from build123d import *

# Parameters (mm, degrees)
BOSS_EXTRUDE1_DEPTH = 3
SKETCH2_R           = 1.6
CUT_EXTRUDE1_DEPTH  = 87.402604127
BOSS_EXTRUDE2_DEPTH = 10
CUT_EXTRUDE2_REACH  = 88.928
SKETCH5_R           = 11.1
CUT_EXTRUDE3_REACH  = 88.928
SKETCH6_R           = 1.3
FILLET1_R           = 1
FILLET2_R           = 4
FILLET3_R           = 4
FILLET4_R           = 2
FILLET5_R           = 2


with BuildPart() as part:
    # Sketch1 → Boss-Extrude1 (new body)
    with BuildSketch(Plane(origin=(0, 0, 0), x_dir=(1, 0, 0), z_dir=(0, 1, 0))):
        Polygon((0, 0), (15, 0), (15, 12.9), (62.1, 12.9), (62.1, 47.1), (15, 47.1), (15, 60), (0, 60), align=None)
    extrude(amount=BOSS_EXTRUDE1_DEPTH)

    # Sketch2 → Cut-Extrude1 (cut, through all)
    with BuildSketch(Plane(origin=(0, 3, 0), x_dir=(1, 0, 0), z_dir=(0, 1, 0))):
        with Locations(Location((7.5, 52.5, 0), (0, 0, 270))):
            Circle(SKETCH2_R)
        with Locations(Location((7.5, 37.5, 0), (0, 0, 270))):
            Circle(SKETCH2_R)
        with Locations(Location((7.5, 7.5, 0), (0, 0, 270))):
            Circle(SKETCH2_R)
        with Locations(Location((7.5, 22.5, 0), (0, 0, 270))):
            Circle(SKETCH2_R)
    extrude(amount=-CUT_EXTRUDE1_DEPTH, mode=Mode.SUBTRACT)

    # Sketch3 → Boss-Extrude2 (add)
    with BuildSketch(Plane(origin=(0, 3, 0), x_dir=(1, 0, 0), z_dir=(0, 1, 0))):
        Polygon((62.1, 12.9), (15, 12.9), (0, 12.9), (0, 15.9), (59.1, 15.9), (59.1, 44.1), (0, 44.1), (0, 47.1), (62.1, 47.1), align=None)
    extrude(amount=BOSS_EXTRUDE2_DEPTH)

    # Sketch5 → Cut-Extrude2 (cut, up to next)
    with BuildSketch(Plane(origin=(0, 3, 0), x_dir=(1, 0, 0), z_dir=(0, 1, 0)), mode=Mode.PRIVATE) as cut_extrude2_sk1:
        with Locations(Location((45, 30, 0), (0, 0, 270))):
            Circle(SKETCH5_R)
    cut_extrude2_tool1 = extrude(cut_extrude2_sk1.sketch, amount=-CUT_EXTRUDE2_REACH, mode=Mode.PRIVATE) & part.part
    add(cut_extrude2_tool1.solids().sort_by_distance((45, 3, -30))[0], mode=Mode.SUBTRACT)

    # Sketch6 → Cut-Extrude3 (cut, up to next)
    with BuildSketch(Plane(origin=(0, 3, 0), x_dir=(1, 0, 0), z_dir=(0, 1, 0)), mode=Mode.PRIVATE) as cut_extrude3_sk1:
        with Locations(Location((56.5, 41.5, 0), (0, 0, 270))):
            Circle(SKETCH6_R)
    cut_extrude3_tool1 = extrude(cut_extrude3_sk1.sketch, amount=-CUT_EXTRUDE3_REACH, mode=Mode.PRIVATE) & part.part
    # Sketch6 → Cut-Extrude3 (cut, up to next)
    with BuildSketch(Plane(origin=(0, 3, 0), x_dir=(1, 0, 0), z_dir=(0, 1, 0)), mode=Mode.PRIVATE) as cut_extrude3_sk2:
        with Locations(Location((33.5, 41.5, 0), (0, 0, 270))):
            Circle(SKETCH6_R)
    cut_extrude3_tool2 = extrude(cut_extrude3_sk2.sketch, amount=-CUT_EXTRUDE3_REACH, mode=Mode.PRIVATE) & part.part
    # Sketch6 → Cut-Extrude3 (cut, up to next)
    with BuildSketch(Plane(origin=(0, 3, 0), x_dir=(1, 0, 0), z_dir=(0, 1, 0)), mode=Mode.PRIVATE) as cut_extrude3_sk3:
        with Locations(Location((33.5, 18.5, 0), (0, 0, 270))):
            Circle(SKETCH6_R)
    cut_extrude3_tool3 = extrude(cut_extrude3_sk3.sketch, amount=-CUT_EXTRUDE3_REACH, mode=Mode.PRIVATE) & part.part
    # Sketch6 → Cut-Extrude3 (cut, up to next)
    with BuildSketch(Plane(origin=(0, 3, 0), x_dir=(1, 0, 0), z_dir=(0, 1, 0)), mode=Mode.PRIVATE) as cut_extrude3_sk4:
        with Locations(Location((56.5, 18.5, 0), (0, 0, 270))):
            Circle(SKETCH6_R)
    cut_extrude3_tool4 = extrude(cut_extrude3_sk4.sketch, amount=-CUT_EXTRUDE3_REACH, mode=Mode.PRIVATE) & part.part
    add(cut_extrude3_tool1.solids().sort_by_distance((56.5, 3, -41.5))[0], mode=Mode.SUBTRACT)
    add(cut_extrude3_tool2.solids().sort_by_distance((33.5, 3, -41.5))[0], mode=Mode.SUBTRACT)
    add(cut_extrude3_tool3.solids().sort_by_distance((33.5, 3, -18.5))[0], mode=Mode.SUBTRACT)
    add(cut_extrude3_tool4.solids().sort_by_distance((56.5, 3, -18.5))[0], mode=Mode.SUBTRACT)

    # Fillet1
    fillet1_edges = [part.edges().sort_by_distance(p)[0] for p in [
        (59.1, 8, -44.1),
        (59.1, 8, -15.9),
    ]]
    fillet(fillet1_edges, radius=FILLET1_R)

    # Fillet2
    fillet2_edges = [part.edges().sort_by_distance(p)[0] for p in [
        (62.1, 6.5, -47.1),
        (62.1, 6.5, -12.9),
    ]]
    fillet(fillet2_edges, radius=FILLET2_R)

    # Fillet3
    fillet3_edges = [part.edges().sort_by_distance(p)[0] for p in [
        (15, 1.5, -47.1),
        (15, 1.5, -12.9),
    ]]
    fillet(fillet3_edges, radius=FILLET3_R)

    # Fillet4
    fillet4_edges = [part.edges().sort_by_distance(p)[0] for p in [
        (9.5, 3, -47.1),
        (9.5, 3, -12.9),
    ]]
    fillet(fillet4_edges, radius=FILLET4_R)

    # Fillet5
    fillet5_edges = [part.edges().sort_by_distance(p)[0] for p in [
        (0, 1.5, -60),
        (15, 1.5, -60),
        (15, 1.5, 0),
        (0, 1.5, 0),
    ]]
    fillet(fillet5_edges, radius=FILLET5_R)


solid = part.part
Source: CAD feature listing. Evaluate the final solid. Frame: model axes, mm. A direction names the side the tool comes from. Coordinates: 2 decimals unless noted, no trailing zeros. Loops run counter-clockwise (first coordinate to the right, second up) from the corner with the lowest first, then second, coordinate; pieces in that order, holes last. Notation, with made-up numbers: (14.25, 75.25) -> (32.25, 75.25) arc R22 ccw to (32.25, 109.25) -> close; hole circle Ø7 at (47.5, -0.75). An arc over 180 degrees is marked (long way). Answer in a Markdown table with one row per item. Add a question column.
Q1. Pull-direction query (Z, two-part tool) for faces 6 (the face through (59.1, 8, -30)), 7 (the face through (8, 1, -60)), 8 (the face through (0, 2, -30)), 9 (the face through (60.897, 6.591, -14.041)); classes: pulls with the +Z half, pulls with the -Z half, needs draft (parallel to the pull), parting line crosses it, or undercut.
Q2. Ray query, line 1 along Z through (x, y) = (24.5, 8.25); line 2 along X through (y, z) = (0.7, -41.5); line 3 along X through (y, z) = (2.3, -7.5). Return the intervals inside material, ascending.
Q3. Reachability of faces 1 (the face through (35, 6, -47.1)), 2 (the face through (7.7, 3, -5.5)), 3 (the face through (8, 3, -55)), 4 (the face through (36, 13, -15)), 5 (the face through (23, 3, -30)) from +Z, -Z, +X, -X, +Y, -Y: full face, straight path, thin tool, end or side. Return the list, or none.
Q4. Contact query for flat-ended pins moving along their axis: pin 1 Ø6 at (x, y) = (41, 5) entering from -Z; pin 2 Ø4 at (x, z) = (56.5, -41.5) entering from +Y; pin 3 Ø1.5 at (y, z) = (6, -43.5) entering from -X; pin 4 Ø1.5 at (y, z) = (3, -13.5) entering from +X. Output: stop coordinate, or through.
Q5. Section A-A on z = -30. Return the cut outline in (x, y), and give its area (3 significant figures).
Q6. Section B-B on x = 7.5. Give the number of separate pieces and of enclosed holes in the cut face, and give its area (3 significant figures).
Q7. Section D-D on y = 6.5. Return the cut outline in (x, z), and give its area (3 significant figures).
Computed values:
| question | item | result |
|---|---|---|
| 1 | face 6 | undercut |
| 1 | face 7 | pulls with the -Z half |
| 1 | face 8 | needs draft |
| 1 | face 9 | pulls with the +Z half |
| 2 | line 1 | z = -47.1 to -44.1, -15.9 to -12.9 |
| 2 | line 2 | x = 0 to 32.2, 34.8 to 55.2, 57.8 to 62.1 |
| 2 | line 3 | x = 0 to 5.9, 9.1 to 15 |
| 3 | face 1 | -Z, +X, +Y |
| 3 | face 2 | +Z, +X, -X, +Y |
| 3 | face 3 | -Z, +X, -X, +Y |
| 3 | face 4 | +Z, -Z, +X, -X, +Y |
| 3 | face 5 | -X, +Y |
| 4 | pin 1 | stops at z = -47.1 |
| 4 | pin 2 | stops at y = 3 |
| 4 | pin 3 | stops at x = 0 |
| 4 | pin 4 | stops at x = 61.1 |
| 5 | outline | (0, 0) -> (33.9, 0) -> (33.9, 3) -> (0, 3) -> close; (56.1, 0) -> (62.1, 0) -> (62.1, 13) -> (59.1, 13) -> (59.1, 3) -> (56.1, 3) -> close |
| 5 | area | 150 mm^2 |
| 6 | separate pieces | 5 |
| 6 | enclosed holes | 0 |
| 6 | area | 203 mm^2 |
| 7 | outline | (0, -47.1) -> (58.1, -47.1) arc R4 ccw to (62.1, -43.1) -> (62.1, -16.9) arc R4 ccw to (58.1, -12.9) -> (0, -12.9) -> (0, -15.9) -> (58.1, -15.9) arc R1 cw to (59.1, -16.9) -> (59.1, -43.1) arc R1 cw to (58.1, -44.1) -> (0, -44.1) -> close |
| 7 | area | 451 mm^2 |
